Work out the finished part from the listing and answer in its coordinate system (mm). A direction names the side the tool comes from. Coordinates: 2 decimals unless noted, no trailing zeros. Order: outer loops, then holes, each group sorted by start corner. A loop starts at its lowest first (then second) coordinate and runs counter-clockwise, first axis right, second up. Notation, with made-up numbers: (-29.5, 74.25) - (-0.5, 74.25) arc R29 ccw to (-0.5, 106.25) - close; hole circle Ø8 at (-35.75, 60). An arc over 180 degrees is marked (long way). Answer as a JSON object with one key per item and string values. Group by question number.
1) Section C-C (x = 36) is taken. Give the vertices of the cut face in (y, z).
2) Section A-A (y = 12.5) is taken. Give the vertices of the cut face in (x, z), plus the area to 3 significant figures.
3) Section D-D (z = 16.5) is taken. Give the vertices of the cut face in (x, y).
4) The mould has two halves that part along X. Classify faces 1 (the face through (29.54, 9.5, 20.94)), 2 (the face through (15, 24, 15)), 3 (the face through (7.71, 13.34, 7.43)), 4 (the face through (0, 13, 7)): released by +X, released by -X, zero draft, split by the parting line, or undercut.
5) Each of these flat-tipped pins is pushed along its axis until it touches: P1, Ø3, axis at x = 32, z = 7.5, coming from the +Y side; P2, Ø5, axis at x = 16.5, y = 11, coming from the +Z side; P3, Ø3, axis at x = 29.5, z = 21, coming from the -Y side. Where does it stop, or does it pass through?
6) Find the intervals of material crossed by line 1 along Z through (x, y) = (32, 19.5); line 2 along X through (y, z) = (21.5, 7.5); line 3 along Y through (x, z) = (20, 20), in increasing order.
7) Section B-B (z = 22.5) is taken. Give the vertices of the cut face in (x, y), plus the area to 3 significant figures.
8) A tool of negligible diameter and unlimited length cuts with its end or side. For faces 5 (the face through (20, 0, 4)), 6 (the face through (40, 12, 7)), 7 (the face through (20, 13, 15)), 8 (the face through (20.66, 5.48, 5.9)), 9 (the face through (8.66, 19.52, 9.1)), from which of +Z, -Z, +X, -X, +Y, -Y can it reach the whole face along a straight path? Write none if from no direction.
Autodesk Inventor part; units mm, degrees
ref_plane "YZ Plane" through (0, 0, 0) normal (1, 0, 0) x (0, 1, 0)
ref_plane "XZ Plane" through (0, 0, 0) normal (0, 1, 0) x (-1, 0, 0)
ref_plane "XY Plane" through (0, 0, 0) normal (0, 0, 1) x (1, 0, 0)
sketch "Sketch1" plane through (0, 0, 0) normal (0, 0, 1) x (1, 0, 0)
  line L0 (0, 0) -> (40, 0)
  line L1 (40, 0) -> (40, 25)
  line L2 (40, 25) -> (0, 25)
  line L3 (0, 25) -> (0, 0)
  dimension "d0" = 40
  dimension "d1" = 25
extrude "Extrusion1" add sketch "Sketch1" along normal blind 15
sketch "Sketch2" plane through (0, 25, 0) normal (0, 1, 0) x (1, 0, 0)
  line L0 (0, 0) -> (0, -15)
  line L1 (0, -7.5) -> (8, -7.5)
  line L2 (40, 0) -> (40, -15)
  line L3 (40, -7.5) -> (32, -7.5)
  dimension "d4" = 8
  dimension "d5" = 8
hole "Hole1" at (8, 25, 7.5) at (32, 25, 7.5) direction (0, -1, 0) diameter 3.4587 depth 10.8 tip angle 118
sketch "Sketch3" plane through (0, 0, 15) normal (0, 0, 1) x (1, 0, 0)
  line L0 (40, 25) -> (0, 25)
  line L1 (20, 25) -> (20, 0) construction
  line L2 (0, 0) -> (40, 0)
  circle A0 centre (20, 12.5) radius 10
  circle A1 centre (20, 12.5) radius 8
  dimension "d13" = 20
extrude "Extrusion2" add sketch "Sketch3" along normal blind 10
sketch "Sketch4" plane through (0, 0, 0) normal (0, -1, 0) x (1, 0, 0)
  line L0 (0, 15) -> (40, 15)
  line L1 (20, 15) -> (20, 0)
  line L2 (40, 0) -> (0, 0)
  point P0 (20, 7.5)
hole "Hole2" at (20, 0, 7.5) direction (0, 1, 0) diameter 3.4587 depth 10.8 tip angle 118
fillet "Fillet1" radius 2 1 edges at (10, 12.5, 15)
sketch "Sketch5" plane through (20, 12.5, 15) normal (0, 0, 1) x (1, 0, 0)
  point P0 (-20, -12.5)
properties part number "charging_port"
Report:
{
 "1": {"outline": "(0, 0) - (25, 0) - (25, 15) - (0, 15) - close"},
 "2": {"outline": "(0, 0) - (40, 0) - (40, 15) - (32, 15) arc R2 cw to (30, 17) - (30, 25) - (28, 25) - (28, 15) - (12, 15) - (12, 25) - (10, 25) - (10, 17) arc R2 cw to (8, 15) - (0, 15) - close", "area": "642 mm²"},
 "3": {"outline": "circle Ø20.13 at (20, 12.5); hole circle Ø16 at (20, 12.5)"},
 "4": {"face 1": "split by the parting line", "face 2": "zero draft", "face 3": "undercut", "face 4": "released by -X"},
 "5": {"P1": "stops at y = 14.06", "P2": "stops at z = 15", "P3": "stops at y = 6.5"},
 "6": {"line 1": "z = 0 to 5.77, 9.23 to 15", "line 2": "x = 0 to 6.27, 9.73 to 30.27, 33.73 to 40", "line 3": "y = 2.5 to 4.5, 20.5 to 22.5"},
 "7": {"outline": "circle Ø20 at (20, 12.5); hole circle Ø16 at (20, 12.5)", "area": "113 mm²"},
 "8": {"face 5": "+Z, -Z, +X, -X, -Y", "face 6": "+Z, -Z, +X, +Y, -Y", "face 7": "+Z", "face 8": "-Y", "face 9": "+Y"}
}
